Here's how the part is built. I have some questions about the finished solid (model axes, mm). Face numbers are marked on the shaded views. A direction names the side the tool comes from. Coordinates: 2 decimals unless noted, no trailing zeros. Write each loop counter-clockwise with the first axis right and the second up, starting at its lowest first coordinate (ties: lowest second). Pieces come first, ordered by that corner, then holes.
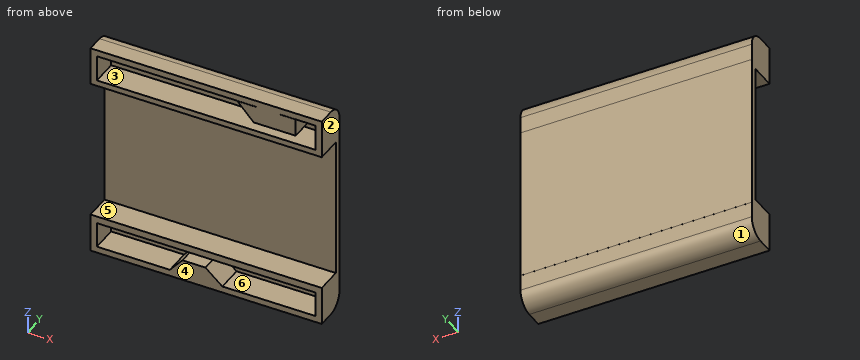
```python
from build123d import *

# Parameters (mm, degrees)
SKETCH_3_W                      = 36
SKETCH_3_H                      = 10
EXTRUDE_1_DEPTH                 = 34
SHELL_1_T                       = -1
EXTRUDE_3_DEPTH                 = 18
EXTRUDE_3_DEPTH_BACK            = 18
SKETCH_4_W                      = 23.985162527
SKETCH_4_H                      = 5.996290528
FILLET_9_R                      = 2.5
EXTRUDE_6_DEPTH                 = 4
EXTRUDE_6_DEPTH_BACK            = 3.2
EXTRUDE_7_DEPTH                 = 4
EXTRUDE_7_DEPTH_BACK            = 3.2
FILLET_11_R                     = 2.5
EXTRUDE_START                   = -5
EXTRUDE_8_DEPTH                 = 9
CUT_EXTRUDE_START               = 17
SKETCH_8_W                      = 9.2
SKETCH_8_H                      = 1.40146724
CUT_EXTRUDE_3_DEPTH             = 0.5
CUT_EXTRUDE_4_REACH             = 40.795
SKETCH_11_W                     = 21.965454815
SKETCH_11_H                     = 3.993719057
CUT_EXTRUDE_4_DIRECTION_2_REACH = 40.795
SKETCH_10_W                     = 1.1
SKETCH_10_H                     = 7.7
SKETCH_10_W_2                   = 1.122304396
SKETCH_10_W_3                   = 1.111152198
SKETCH_10_W_4                   = 1.088342312
SKETCH_10_W_5                   = 1.094171156
CUT_EXTRUDE_5_DEPTH             = 0.991590454
SPLIT_START                     = -5
SPLIT_BODIES_2_OUTLINE_W        = 36
SPLIT_BODIES_2_OUTLINE_H        = 34
SPLIT_BODIES_2_OUTLINE_W_2      = 1.1
SPLIT_BODIES_2_OUTLINE_H_2      = 7.7
SPLIT_BODIES_2_OUTLINE_W_3      = 1.111152198
SPLIT_BODIES_2_OUTLINE_W_4      = 1.094171156
SPLIT_BODIES_2_OUTLINE_W_5      = 1.122304396
SPLIT_BODIES_2_OUTLINE_W_6      = 1.088342312
SPLIT_BODIES_2_DEPTH            = 4.942187478


# Read off the part's stored shape, not the designer's step: 分割1, 分割2
with BuildPart() as part:
    # 草图3 → 凸台-拉伸1 (new body)
    with BuildSketch(Plane.XY):
        Rectangle(SKETCH_3_W, SKETCH_3_H)
    extrude(amount=EXTRUDE_1_DEPTH)

    # 抽壳1
    shell_1_openings = [part.faces().sort_by_distance(p)[0] for p in [
        (0, -5, 17),
    ]]
    offset(amount=SHELL_1_T, openings=shell_1_openings, kind=Kind.INTERSECTION)

    # 草图4 → 凸台-拉伸3 (add, two sides: drawn at the far end of the back side and taken through both)
    with BuildSketch(Plane(origin=(0, 0, 0), x_dir=(0, 0, -1), z_dir=(1, 0, 0)).offset(-EXTRUDE_3_DEPTH_BACK)):
        with Locations((-16.943109173, 2.00655481)):
            Rectangle(SKETCH_4_W, SKETCH_4_H)
    extrude(amount=EXTRUDE_3_DEPTH + EXTRUDE_3_DEPTH_BACK)

    # 圆角9
    fillet_9_edges = [part.edges().sort_by_distance(p)[0] for p in [
        (0, 5, 34),
    ]]
    fillet(fillet_9_edges, radius=FILLET_9_R)

    # 草图6 → 凸台-拉伸6 (add, two sides: drawn at the far end of the back side and taken through both)
    with BuildSketch(Plane(origin=(0, 0, 0), x_dir=(1, 0, 0), z_dir=(0, 1, 0)).offset(-EXTRUDE_6_DEPTH_BACK)):
        Polygon((4.859681811, -32.9683063), (7.403408748, -30.245536487), (12.359177608, -30.245536487), (13.940012235, -30.245536487), (13.940012235, -32.9683063), align=None)
    extrude(amount=EXTRUDE_6_DEPTH + EXTRUDE_6_DEPTH_BACK)

    # 草图7 → 凸台-拉伸7 (add, two sides: drawn at the far end of the back side and taken through both)
    with BuildSketch(Plane(origin=(0, 0, 0), x_dir=(1, 0, 0), z_dir=(0, 1, 0)).offset(-EXTRUDE_7_DEPTH_BACK)):
        Polygon((2.54458171, -0.980815803), (-0.105019187, -3.27043557), (-3.683509766, -3.27043557), (-5.662056301, -0.980815803), align=None)
    extrude(amount=EXTRUDE_7_DEPTH + EXTRUDE_7_DEPTH_BACK)

    # 圆角11
    fillet_11_edges = [part.edges().sort_by_distance(p)[0] for p in [
        (0, 5, 0),
    ]]
    fillet(fillet_11_edges, radius=FILLET_11_R)

    # 草图5 → 凸台-拉伸8 (add)
    with BuildSketch(Plane(origin=(0, 0, 0), x_dir=(1, 0, 0), z_dir=(0, 1, 0)).offset(EXTRUDE_START)):
        Polygon((-3.212354085, -1), (-2.299075535, -1.958092867), (-1.257675535, -1.958092867), (-0.046128087, -1), align=None)
        Polygon((7.806276899, -33), (8.868785029, -31.937293749), (11.523785029, -31.937293749), (11.523785029, -33), align=None)
    extrude(amount=EXTRUDE_8_DEPTH)

    # 草图8 → 切除-拉伸3 (cut)
    with BuildSketch(Plane(origin=(0, 0, 0), x_dir=(0, 0, -1), z_dir=(1, 0, 0)).offset(CUT_EXTRUDE_START)):
        with Locations((-26.021321233, -4.299270344)):
            Rectangle(SKETCH_8_W, SKETCH_8_H)
    extrude(amount=CUT_EXTRUDE_3_DEPTH, mode=Mode.SUBTRACT)

    # 切除-拉伸4: up to this face of the body (flat: up to its plane)
    cut_extrude_4_end = Plane(part.part.faces().sort_by_distance((-18, -0.033638706, 16.999980993))[0])
    # 草图11 → 切除-拉伸4 (cut, up to the picked face)
    with BuildSketch(Plane(origin=(0, 0, 0), x_dir=(0, 0, -1), z_dir=(1, 0, 0)), mode=Mode.PRIVATE) as cut_extrude_4_sk1:
        with Locations((-17.041422709, 1.939047007)):
            Rectangle(SKETCH_11_W, SKETCH_11_H)
    cut_extrude_4_tool1 = split(extrude(cut_extrude_4_sk1.sketch, amount=-CUT_EXTRUDE_4_REACH, mode=Mode.PRIVATE), bisect_by=cut_extrude_4_end, keep=Keep.BOTH, mode=Mode.PRIVATE)
    add(cut_extrude_4_tool1.solids().sort_by(Axis((0, 1.939047, 17.041423), (-1, 0, 0)))[0], mode=Mode.SUBTRACT)

    # 切除-拉伸4 direction 2: up to this face of the body (flat: up to its plane)
    cut_extrude_4_direction_2_end = Plane(part.part.faces().sort_by_distance((18, -0.033638706, 16.999980993))[0])
    # 草图11 → 切除-拉伸4 direction 2 (cut, up to the picked face)
    with BuildSketch(Plane(origin=(0, 0, 0), x_dir=(0, 0, -1), z_dir=(1, 0, 0)), mode=Mode.PRIVATE) as cut_extrude_4_direction_2_sk1:
        with Locations((-17.041422709, 1.939047007)):
            Rectangle(SKETCH_11_W, SKETCH_11_H)
    cut_extrude_4_direction_2_tool1 = split(extrude(cut_extrude_4_direction_2_sk1.sketch, amount=CUT_EXTRUDE_4_DIRECTION_2_REACH, mode=Mode.PRIVATE), bisect_by=cut_extrude_4_direction_2_end, keep=Keep.BOTH, mode=Mode.PRIVATE)
    add(cut_extrude_4_direction_2_tool1.solids().sort_by(Axis((0, 1.939047, 17.041423), (1, 0, 0)))[0], mode=Mode.SUBTRACT)

    # 草图10 → 切除-拉伸5 (cut)
    with BuildSketch(Plane(origin=(0, 0, 0), x_dir=(1, 0, 0), z_dir=(0, 1, 0))):
        with Locations((-10.631432442, -10.52972417)):
            Rectangle(SKETCH_10_W, SKETCH_10_H)
        with Locations((-10.631432442, -20.605915071)):
            Rectangle(SKETCH_10_W, SKETCH_10_H)
        with Locations((10.829939073, -20.605915071)):
            Rectangle(SKETCH_10_W, SKETCH_10_H)
        with Locations((10.829939073, -10.52972417)):
            Rectangle(SKETCH_10_W, SKETCH_10_H)
        with Locations((-6.938026669, -10.52972417)):
            Rectangle(SKETCH_10_W_2, SKETCH_10_H)
        with Locations((-6.943602768, -20.605915071)):
            Rectangle(SKETCH_10_W_3, SKETCH_10_H)
        with Locations((7.321076066, -10.52972417)):
            Rectangle(SKETCH_10_W_4, SKETCH_10_H)
        with Locations((7.323990488, -20.605915071)):
            Rectangle(SKETCH_10_W_5, SKETCH_10_H)
    extrude(amount=-CUT_EXTRUDE_5_DEPTH, mode=Mode.SUBTRACT)


with BuildPart() as body_2:
    # Split Bodies 1: the piece on the far side of the plane
    add(part.part)
    split(bisect_by=Plane(origin=(0, -0.057812522, 0), x_dir=(1, 0, 0), z_dir=(0, 1, 0)), keep=Keep.BOTTOM)

    # Split Bodies 2 outline → Split Bodies 2 (cut)
    with BuildSketch(Plane(origin=(0, 0, 0), x_dir=(1, 0, 0), z_dir=(0, 1, 0)).offset(SPLIT_START)):
        with Locations((0, -17)):
            Rectangle(SPLIT_BODIES_2_OUTLINE_W, SPLIT_BODIES_2_OUTLINE_H)
        Polygon((-17, -28.935690436), (17, -28.935690436), (17, -33), (11.523785029, -33), (11.523785029, -32.9683063), (13.940012235, -32.9683063), (13.940012235, -30.245536487), (7.403408748, -30.245536487), (4.859681811, -32.9683063), (7.83796469, -32.9683063), (7.806276899, -33), (-17, -33), align=None, mode=Mode.SUBTRACT)
        Polygon((17, -4.950527909), (-17, -4.950527909), (-17, -1), (-5.645478515, -1), (-3.683509766, -3.27043557), (-0.105019187, -3.27043557), (2.522381315, -1), (17, -1), align=None, mode=Mode.SUBTRACT)
        with Locations((-10.631432442, -20.605915071)):
            Rectangle(SPLIT_BODIES_2_OUTLINE_W_2, SPLIT_BODIES_2_OUTLINE_H_2, mode=Mode.SUBTRACT)
        with Locations((-6.943602768, -20.605915071)):
            Rectangle(SPLIT_BODIES_2_OUTLINE_W_3, SPLIT_BODIES_2_OUTLINE_H_2, mode=Mode.SUBTRACT)
        with Locations((7.323990488, -20.605915071)):
            Rectangle(SPLIT_BODIES_2_OUTLINE_W_4, SPLIT_BODIES_2_OUTLINE_H_2, mode=Mode.SUBTRACT)
        with Locations((10.829939073, -20.605915071)):
            Rectangle(SPLIT_BODIES_2_OUTLINE_W_2, SPLIT_BODIES_2_OUTLINE_H_2, mode=Mode.SUBTRACT)
        with Locations((-10.631432442, -10.52972417)):
            Rectangle(SPLIT_BODIES_2_OUTLINE_W_2, SPLIT_BODIES_2_OUTLINE_H_2, mode=Mode.SUBTRACT)
        with Locations((-6.938026669, -10.52972417)):
            Rectangle(SPLIT_BODIES_2_OUTLINE_W_5, SPLIT_BODIES_2_OUTLINE_H_2, mode=Mode.SUBTRACT)
        with Locations((7.321076066, -10.52972417)):
            Rectangle(SPLIT_BODIES_2_OUTLINE_W_6, SPLIT_BODIES_2_OUTLINE_H_2, mode=Mode.SUBTRACT)
        with Locations((10.829939073, -10.52972417)):
            Rectangle(SPLIT_BODIES_2_OUTLINE_W_2, SPLIT_BODIES_2_OUTLINE_H_2, mode=Mode.SUBTRACT)
    extrude(amount=SPLIT_BODIES_2_DEPTH, mode=Mode.SUBTRACT)


with BuildPart() as part_1:
    add(part.part)

    # Split Bodies 1
    split(bisect_by=Plane(origin=(0, -0.057812522, 0), x_dir=(1, 0, 0), z_dir=(0, 1, 0)), keep=Keep.TOP)


solid = part_1.part
```
1) On a 3-axis mill with a long thin cutter (end or side, diameter ignored), from which of +Z, -Z, +X, -X, +Y, -Y can I reach the whole of each face in a straight line? I mean the marked faces 4, 5 and 6. Say none if no direction works.
Values follow:
face 4: +Z, -Z, +X, -X, -Y
face 5: +X, -X, -Y
face 6: -Y
2) Imagine slicing it at D-D on y = 4.4. Please give me the cut outline in (x, z), then the cut area to 3 significant figures.
Values follow:
outline: (-18, 0.88) - (18, 0.88) - (18, 33.12) - (-18, 33.12) - close
area: 1,160 mm2
3) Will these pins go through, and if not, where does the flat tip stop? pin 1 (2 mm diameter, centred on x = -0.5, z = 30.5, fed in from -Y); pin 2 (1.3 mm diameter, centred on x = -0.5, z = 30.5, fed in from +Y).
Values follow:
pin 1: stops at y = 4
pin 2: stops at y = 5
4) Imagine slicing it at C-C on z = 16. Please give me the cut outline in (x, y), then the cut area to 3 significant figures.
Values follow:
outline: (-18, 3.94) - (18, 3.94) - (18, 5) - (-18, 5) - close
area: 38.5 mm2
5) We'd pull the mould along X, two halves only. Please class the marked faces 1, 2 and 3: pulls with the +X half, pulls with the -X half, needs draft (parallel to the pull), parting line crosses it, or undercut.
Values follow:
face 1: needs draft
face 2: pulls with the +X half
face 3: undercut
6) Imagine slicing it at A-A on y = 1.95. Count the separate pieces of the cut face and the enclosed holes in it, then the cut area to 3 significant figures.
Values follow:
separate pieces: 2
enclosed holes: 2
area: 195 mm2
7) I need wall thicknesses on probe 1 along Z at (x, y) = (-9, 2.35); probe 2 along Z at (x, y) = (-0.5, 0.55); probe 3 along X at (y, z) = (3.2, 32). Which ranges of each line are inside material? Lowest first, please.
Values follow:
probe 1: z = 0 to 1, 4.95 to 6.06, 28.02 to 28.94, 33 to 34
probe 2: z = 0 to 3.27, 4.95 to 6.06, 28.02 to 28.94, 33 to 34
probe 3: x = -18 to -17, 5.76 to 13.94, 17 to 18
